from build123d import *

# Parameters (mm, degrees)
F3_D = 10
F4_R = 5
F6_D = 7


with BuildPart() as f1:
    # F0 (on Front) → F1 (revolve)
    with BuildSketch(Plane.XZ):
        Polygon((0, 5), (0, 0), (14, 0), (14, 5), (9.5, 5), (9.5, 20.154822), (14, 20.154822), (14, 26.396757), (0, 26.396757), (0, 20.154822), (4.5, 20.154822), (4.5, 5), align=None)
    revolve(axis=Axis((7, 0, 0), (1, 0, 0)))

    # F3 (through all)
    with Locations(Plane.YZ.offset(9.5)):
        with Locations((0, 12.574399), (-11.958964, 3.885703), (-7.391046, -10.172902), (7.391046, -10.172902), (11.958964, 3.885703)):
            Hole(F3_D / 2)

    # F4
    f4_edges = [f1.edges().sort_by_distance(p)[0] for p in [
        (14, 0, -26.396757),
        (0, 0, -26.396757),
    ]]
    fillet(f4_edges, radius=F4_R)

    # F6 (through all)
    with Locations(Plane.YZ.offset(14)):
        with Locations((0, 0)):
            Hole(F6_D / 2)


solid = f1.part
Input: part model. Units: mm. Frame: model coordinates. A direction names the side the tool comes from. Coordinates: 2 decimals unless noted, no trailing zeros. Write each loop counter-clockwise with the first axis right and the second up, starting at its lowest first coordinate (ties: lowest second). Pieces come first, ordered by that corner, then holes. Notation, with made-up numbers: M -29,57 L -5,57 A36 cw -5,92 Z; hole C -23,-18 d9. An arc over 180 degrees is marked long. Answer as a JSON object with one key per item and string values. Group by question number.
(1) Section B-B on x = 11.25. Output: boundary loops of the cut face in (y, z).
(2) Set-up query: faces 1 (the face through (2.282, 19.676, -4.369)), 2 (the face through (9.5, 4, -4)), 3 (the face through (6.965, 15.927, 0.843)). Return all of +Z, -Z, +X, -X, +Y, -Y with unobstructed straight access to the full face (end or side cutting, diameter ignored); none if empty.
(3) Ray query, line 1 along Y through (x, z) = (5, -13); line 2 along Z through (x, y) = (12.35, 0); line 3 along Z through (x, y) = (10.75, -4). Return the intervals inside material, ascending. Write a range as [from, to].
(4) Section A-A on y = 0. Give the number of separate pieces and of enclosed holes in the cut face, plus the area to 3 significant figures.
(5) Mould query, pull axis Y, two halves, no side actions, for faces 4 (the face through (6.97, -26.17, -3.44)), 5 (the face through (0, 3.3, 2.2)), 6 (the face through (6.965, 1.084, 7.693)). Classes: pulls with the +Y half, pulls with the -Y half, needs draft (parallel to the pull), parting line crosses it, or undercut.
(6) Contact query for flat-ended pins moving along their axis: P1, Ø8, axis at y = 7.39, z = -10.17, coming from the -X side; P2, Ø8, axis at x = 7.5, y = -20, coming from the -Z side (3 decimals); P3, Ø2, axis at y = 1.5, z = -14, coming from the +X side; P4, Ø6, axis at x = 4.5, y = 6.5, coming from the +Z side. Output: stop coordinate, or through.
(7) Section C-C on x = 8. Output: boundary loops of the cut face in (y, z), plus the area to 3 significant figures.
Result set:
{
 "1": {"outline": "C 0,0 d51.72; C 0,0 d10; hole C 0,0 d40.31; hole C 0,0 d7"},
 "2": {"face 1": "-X", "face 2": "+X", "face 3": "+X, -X"},
 "3": {"line 1": "y = [-22.97, -11.52], [-3.27, 3.27], [11.52, 22.97]", "line 2": "z = [-25.11, -20.15], [-5, -3.5], [3.5, 5], [20.15, 25.11]", "line 3": "z = [-25.77, -19.75], [-3, 3], [19.75, 25.77]"},
 "4": {"separate pieces": "3", "enclosed holes": "0", "area": "297 mm2"},
 "5": {"face 4": "parting line crosses it", "face 5": "needs draft", "face 6": "undercut"},
 "6": {"P1": "passes through", "P2": "stops at z = -20.995", "P3": "stops at x = 9.5", "P4": "stops at z = 26.16"},
 "7": {"outline": "C 0,0 d52.79; hole C -11.96,3.89 d10; hole C -7.39,-10.17 d10; hole C 0,12.57 d10; hole C 0,0 d7; hole C 7.39,-10.17 d10; hole C 11.96,3.89 d10", "area": "1,760 mm2"}
}
